Here's how the part is built. I have some questions about the finished solid (model axes, mm). Face numbers are marked on the shaded views. Coordinates: 2 decimals unless noted, no trailing zeros. Loops run counter-clockwise (first coordinate to the right, second up) from the corner with the lowest first, then second, coordinate; pieces in that order, holes last. Notation, with made-up numbers: (64.5, 68.25) -> (72.5, 68.25) arc R25 cw to (72.5, 81.25) -> close; hole circle Ø6 at (61, -18). An arc over 180 degrees is marked (long way). Answer as a JSON object with one key per item and string values. Group by question number.
Q1. I want a section at A-A on y = 44. Write out the boundary of the cut face in (x, z).
Q2. I want a section at C-C on z = 2.5. Count the separate pieces of the cut face and the enclosed holes in it, then the cut area to 3 significant figures.
Q3. I want a section at D-D on x = 10. Write out the boundary of the cut face in (y, z), then the cut area to 3 significant figures.
Q4. I'm going to push flat-ended pins straight in: pin 1 (2.5 mm diameter, centred on x = 64, z = 2.5, fed in from +Y); pin 2 (1.5 mm diameter, centred on y = 89.5, z = 3.5, fed in from -X); pin 3 (4 mm diameter, centred on y = 129.5, z = 2.5, fed in from -X). Where does each tip first touch, or does it pass through?
Q5. I want a section at B-B on x = 77. Write out the boundary of the cut face in (y, z).
Q6. I need wall thicknesses on line 1 (X direction, y = 109, z = 4); line 2 (Y direction, x = 27.56, z = 7.7); line 3 (Y direction, x = 66, z = 2). Which ranges of each line are inside material? Lowest first, please.
Q7. Thinking about a two-plate mould opening in Y: for the marked faces 1 and 2, which applies, released by +Y, released by -Y, zero draft, split by the parting line, or undercut?
```python
from build123d import *

# Parameters (mm, degrees)
SKETCH1_R           = 3.25
SKETCH1_R_2         = 1.45
SKETCH1_R_3         = 0.95
SKETCH1_W           = 52.44
SKETCH1_H           = 43
BOSS_EXTRUDE1_DEPTH = 5
SKETCH2_R           = 5
SKETCH2_R_2         = 1.45
BOSS_EXTRUDE2_DEPTH = 2
SKETCH3_R           = 3
SKETCH3_R_2         = 0.945605266
SKETCH3_R_3         = 0.976454059
SKETCH3_R_4         = 0.939469919
SKETCH3_R_5         = 0.95
BOSS_EXTRUDE3_DEPTH = 5


with BuildPart() as part:
    # Sketch1 → Boss-Extrude1 (new body)
    with BuildSketch(Plane.XY):
        with BuildLine():
            Line((-5.367112971, 5.238711517), (22.56, 33.850321407))
            Line((22.56, 33.850321407), (22.56, 114))
            Line((22.56, 114), (30.283459854, 142.689687483))
            ThreePointArc((30.283459854, 142.689687483), (36.56, 147.5), (42.836540146, 142.689687483))
            Line((42.836540146, 142.689687483), (50.56, 114))
            Line((50.56, 114), (91, 114))
            Line((91, 114), (91, 18.850321407))
            Line((91, 18.850321407), (97.880809624, 2.984034001))
            ThreePointArc((97.880809624, 2.984034001), (97.517806061, -3.71055308), (91.9464361, -7.440044268))
            Line((91.9464361, -7.440044268), (32.8309574, -14.960029512))
            ThreePointArc((32.8309574, -14.960029512), (31.949174794, -14.993704709), (31.075204637, -14.871841068))
            Line((31.075204637, -14.871841068), (-1.687193044, -7.307761602))
            ThreePointArc((-1.687193044, -7.307761602), (-7.196826055, -2.11085166), (-5.367112971, 5.238711517))
        make_face()
        Circle(SKETCH1_R, mode=Mode.SUBTRACT)
        with Locations((91, 0)):
            Circle(SKETCH1_R, mode=Mode.SUBTRACT)
        with Locations((32.2, -10)):
            Circle(SKETCH1_R_2, mode=Mode.SUBTRACT)
        with Locations((83.7, 22.7)):
            Circle(SKETCH1_R_2, mode=Mode.SUBTRACT)
        with Locations((27.56, 109)):
            Circle(SKETCH1_R_3, mode=Mode.SUBTRACT)
        with Locations((27.56, 60)):
            Circle(SKETCH1_R_3, mode=Mode.SUBTRACT)
        with Locations((85.56, 60)):
            Circle(SKETCH1_R_3, mode=Mode.SUBTRACT)
        with Locations((85.56, 109)):
            Circle(SKETCH1_R_3, mode=Mode.SUBTRACT)
        with BuildLine():
            Line((33.273349419, 41.853300017), (85, 27.444671021))
            Line((85, 27.444671021), (85, 55))
            Line((85, 55), (32.56, 55))
            Line((32.56, 55), (32.56, 41.983767061))
            ThreePointArc((32.56, 41.983767061), (32.919637445, 41.934732767), (33.273349419, 41.853300017))
        make_face(mode=Mode.SUBTRACT)
        with Locations((56.78, 84.5)):
            Rectangle(SKETCH1_W, SKETCH1_H, mode=Mode.SUBTRACT)
        Polygon((32.2, -6), (5, 0), (32.2, 27.866675292), (84.517456272, 13.293475424), (86, 0), align=None, mode=Mode.SUBTRACT)
        with BuildLine():
            Line((38.06, 141), (38.06, 123))
            ThreePointArc((38.06, 123), (36.56, 121.5), (35.06, 123))
            Line((35.06, 123), (35.06, 141))
            ThreePointArc((35.06, 141), (36.56, 142.5), (38.06, 141))
        make_face(mode=Mode.SUBTRACT)
    extrude(amount=BOSS_EXTRUDE1_DEPTH)

    # Sketch2 → Boss-Extrude2 (add)
    with BuildSketch(Plane.XY.offset(5)):
        with Locations((83.7, 22.7)):
            Circle(SKETCH2_R)
        with Locations((83.7, 22.7)):
            Circle(SKETCH2_R_2, mode=Mode.SUBTRACT)
        with BuildLine():
            Line((32.2, -6), (34.773281255, -5.71301696))
            ThreePointArc((34.773281255, -5.71301696), (31.991216079, -14.995639026), (29.993401427, -5.513250315))
            Line((29.993401427, -5.513250315), (32.2, -6))
        make_face()
        with Locations((32.2, -10)):
            Circle(SKETCH2_R_2, mode=Mode.SUBTRACT)
    extrude(amount=BOSS_EXTRUDE2_DEPTH)

    # Sketch3 → Boss-Extrude3 (add)
    with BuildSketch(Plane.XY.offset(5)):
        with Locations((27.56, 60)):
            Circle(SKETCH3_R)
        with Locations((27.56, 60)):
            Circle(SKETCH3_R_2, mode=Mode.SUBTRACT)
        with Locations((85.56, 60)):
            Circle(SKETCH3_R)
        with Locations((85.56, 60)):
            Circle(SKETCH3_R_3, mode=Mode.SUBTRACT)
        with Locations((85.56, 109)):
            Circle(SKETCH3_R)
        with Locations((85.56, 109)):
            Circle(SKETCH3_R_4, mode=Mode.SUBTRACT)
        with Locations((27.56, 109)):
            Circle(SKETCH3_R)
        with Locations((27.56, 109)):
            Circle(SKETCH3_R_5, mode=Mode.SUBTRACT)
    extrude(amount=BOSS_EXTRUDE3_DEPTH)


solid = part.part
```
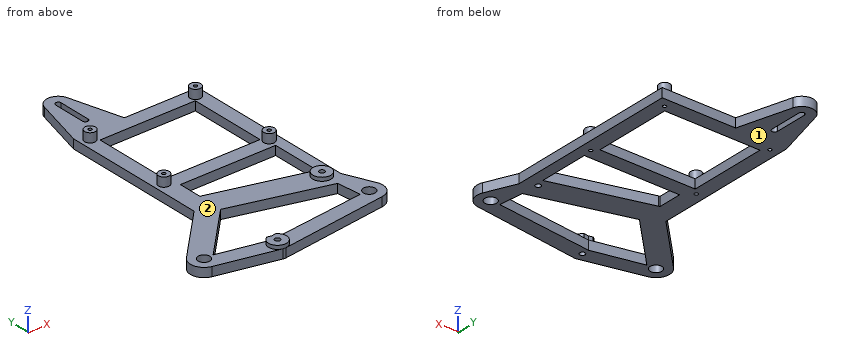
Result set:
{
 "1": {"outline": "(22.56, 0) -> (32.56, 0) -> (32.56, 5) -> (22.56, 5) -> close; (85, 0) -> (91, 0) -> (91, 5) -> (85, 5) -> close"},
 "2": {"separate pieces": "1", "enclosed holes": "12", "area": "5,000 mm²"},
 "3": {"outline": "(-10.01, 0) -> (-1.1, 0) -> (-1.1, 5) -> (-10.01, 5) -> close; (5.12, 0) -> (20.98, 0) -> (20.98, 5) -> (5.12, 5) -> close", "area": "124 mm²"},
 "4": {"pin 1": "stops at y = 114", "pin 2": "stops at x = 22.56", "pin 3": "stops at x = 26.19"},
 "5": {"outline": "(-9.34, 0) -> (-1, 0) -> (-1, 5) -> (-9.34, 5) -> close; (15.39, 0) -> (29.67, 0) -> (29.67, 5) -> (15.39, 5) -> close; (55, 0) -> (63, 0) -> (63, 5) -> (55, 5) -> close; (106, 0) -> (114, 0) -> (114, 5) -> (106, 5) -> close"},
 "6": {"line 1": "x = 22.56 to 26.61, 28.51 to 84.61, 86.51 to 91", "line 2": "y = 57 to 59.05, 60.95 to 63, 106 to 108.05, 109.95 to 112", "line 3": "y = -10.74 to -2.23, 18.45 to 32.74, 55 to 63, 106 to 114"},
 "7": {"face 1": "zero draft", "face 2": "undercut"}
}
